Here's how the part is built. I have some questions about the finished solid (model axes, mm). Coordinates: 2 decimals unless noted, no trailing zeros. Write each loop counter-clockwise with the first axis right and the second up, starting at its lowest first coordinate (ties: lowest second). Pieces come first, ordered by that corner, then holes.
Item 1: If we section it at C-C (z = 0.7): Count the separate pieces of the cut face and the enclosed holes in it, then the cut area to 3 significant figures.
Item 2: If we section it at B-B (x = 34.5): Please give me the cut outline in (y, z).
Item 3: If we section it at A-A (y = -21.5): Please give me the cut outline in (x, z).
Item 4: I'm going to push a flat-ended pin straight in: pin 1 Ø4 at (x, y) = (-4, -4.5) entering from +Z. Where does the tip first touch, or does it pass through?
Item 5: If I drill on line 1 (X direction, y = -25, z = 3.65); line 2 (X direction, y = 7.5, z = 2.3); line 3 (Y direction, x = 62, z = 0.25), over which ranges is the centre line in solid material (lowest first)?
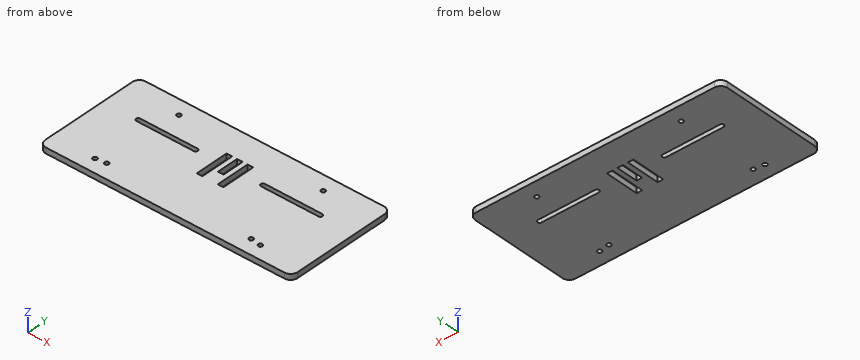
from build123d import *

# Parameters (mm, degrees)
SKETCH1_W           = 180
SKETCH1_H           = 80
SKETCH1_R           = 1.5
BOSS_EXTRUDE1_DEPTH = 4
SKETCH2_W           = 4
SKETCH2_H           = 24
SKETCH2_H_2         = 15.4
CUT_EXTRUDE1_DEPTH  = 4
FILLET1_R           = 5


with BuildPart() as part:
    # Sketch1 → Boss-Extrude1 (new body)
    with BuildSketch(Plane.XY):
        with Locations((2.700642055, -21.117125984)):
            Rectangle(SKETCH1_W, SKETCH1_H)
        with Locations((61.700642055, -51.117125984)):
            Circle(SKETCH1_R, mode=Mode.SUBTRACT)
        with Locations((-56.299357945, -51.117125984)):
            Circle(SKETCH1_R, mode=Mode.SUBTRACT)
        with Locations((-48.799357945, 7.882874016)):
            Circle(SKETCH1_R, mode=Mode.SUBTRACT)
        with Locations((54.200642055, 7.882874016)):
            Circle(SKETCH1_R, mode=Mode.SUBTRACT)
        with Locations((54.200642055, -50.117125984)):
            Circle(SKETCH1_R, mode=Mode.SUBTRACT)
        with Locations((-48.799357945, -50.117125984)):
            Circle(SKETCH1_R, mode=Mode.SUBTRACT)
        with BuildLine():
            Line((-62.299357945, -8.117125984), (-21.299357945, -8.117125984))
            ThreePointArc((-21.299357945, -8.117125984), (-19.799357945, -9.617125984), (-21.299357945, -11.117125984))
            Line((-21.299357945, -11.117125984), (-62.299357945, -11.117125984))
            ThreePointArc((-62.299357945, -11.117125984), (-63.799357945, -9.617125984), (-62.299357945, -8.117125984))
        make_face(mode=Mode.SUBTRACT)
        with BuildLine():
            Line((26.700642055, -8.117125984), (67.700642055, -8.117125984))
            ThreePointArc((67.700642055, -8.117125984), (69.200642055, -9.617125984), (67.700642055, -11.117125984))
            Line((67.700642055, -11.117125984), (26.700642055, -11.117125984))
            ThreePointArc((26.700642055, -11.117125984), (25.200642055, -9.617125984), (26.700642055, -8.117125984))
        make_face(mode=Mode.SUBTRACT)
    extrude(amount=BOSS_EXTRUDE1_DEPTH)

    # Sketch2 → Cut-Extrude1 (cut)
    with BuildSketch(Plane.XY.offset(4)):
        with Locations((-4.799357945, -13.117125984)):
            Rectangle(SKETCH2_W, SKETCH2_H)
        with Locations((2.700642055, -8.817125984)):
            Rectangle(SKETCH2_W, SKETCH2_H_2)
        with Locations((10.200642055, -13.117125984)):
            Rectangle(SKETCH2_W, SKETCH2_H)
    extrude(amount=-CUT_EXTRUDE1_DEPTH, mode=Mode.SUBTRACT)

    # Fillet1
    fillet1_edges = [part.edges().sort_by_distance(p)[0] for p in [
        (-87.299357945, 18.882874016, 2),
        (92.700642055, 18.882874016, 2),
        (92.700642055, -61.117125984, 2),
        (-87.299357945, -61.117125984, 2),
    ]]
    fillet(fillet1_edges, radius=FILLET1_R)


solid = part.part
Answer list:
1. separate pieces: 1
1. enclosed holes: 11
1. area: 13,800 mm2
2. outline: (-61.12, 0) - (-11.12, 0) - (-11.12, 4) - (-61.12, 4) - close; (-8.12, 0) - (18.88, 0) - (18.88, 4) - (-8.12, 4) - close
3. outline: (-87.3, 0) - (-6.8, 0) - (-6.8, 4) - (-87.3, 4) - close; (-2.8, 0) - (8.2, 0) - (8.2, 4) - (-2.8, 4) - close; (12.2, 0) - (92.7, 0) - (92.7, 4) - (12.2, 4) - close
4. pin 1: stops at z = 4
5. line 1: x = -87.3 to -6.8, -2.8 to 8.2, 12.2 to 92.7
5. line 2: x = -87.3 to -50.25, -47.35 to 52.75, 55.65 to 92.7
5. line 3: y = -61.12 to -52.59, -49.65 to -11.12, -8.12 to 18.88
